from build123d import *

# Parameters (mm, degrees)
SKETCH1_R           = 14.125
BOSS_EXTRUDE1_DEPTH = 1.55
BOSS_EXTRUDE2_DEPTH = 1.55
SKETCH4_R           = 1.75
BOSS_EXTRUDE3_DEPTH = 9
CUT_EXTRUDE1_REACH  = 28.959
SKETCH5_R           = 4.75


with BuildPart() as part:
    # Sketch1 → Boss-Extrude1 (new body)
    with BuildSketch(Plane.XY):
        with Locations(Location((0, 0, 0), (0, 0, 180))):
            Circle(SKETCH1_R)
    extrude(amount=BOSS_EXTRUDE1_DEPTH)

    # Sketch2 → Boss-Extrude2 (add)
    with BuildSketch(Plane.XY):
        with BuildLine():
            Line((-17.5, 3.625), (17.5, 3.625))
            ThreePointArc((17.5, 3.625), (21.125, 0), (17.5, -3.625))
            Line((17.5, -3.625), (-17.5, -3.625))
            ThreePointArc((-17.5, -3.625), (-21.125, 0), (-17.5, 3.625))
        make_face()
    extrude(amount=BOSS_EXTRUDE2_DEPTH)

    # Sketch4 → Boss-Extrude3 (add)
    with BuildSketch(Plane.XY):
        with Locations((-17.5, 0)):
            Circle(SKETCH4_R)
        with Locations((17.5, 0)):
            Circle(SKETCH4_R)
    extrude(amount=BOSS_EXTRUDE3_DEPTH)

    # Sketch5 → Cut-Extrude1 (cut, up to next)
    with BuildSketch(Plane(origin=(0, 0, 0), x_dir=(-1, 0, 0), z_dir=(0, 0, -1)), mode=Mode.PRIVATE) as cut_extrude1_sk1:
        with Locations((0, 8)):
            Circle(SKETCH5_R)
    cut_extrude1_tool1 = extrude(cut_extrude1_sk1.sketch, amount=-CUT_EXTRUDE1_REACH, mode=Mode.PRIVATE) & part.part
    add(cut_extrude1_tool1.solids().sort_by_distance((0, 8, 0))[0], mode=Mode.SUBTRACT)


solid = part.part
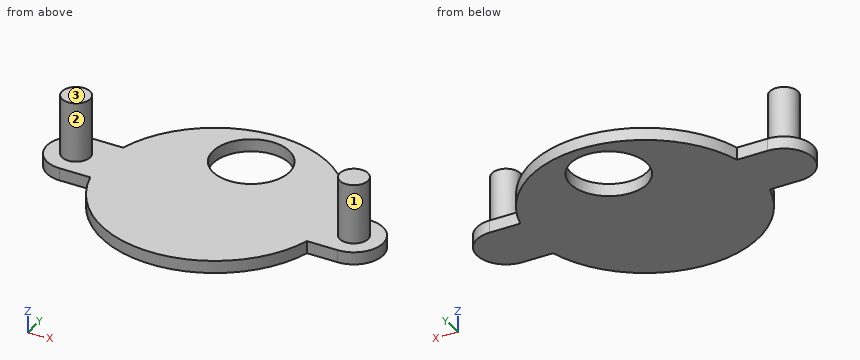
Part model, mm, in its own coordinate system. Face numbers are marked on the shaded views. Give positions to 0.01 mm unless a question says otherwise; leave off trailing zeros. Loops run counter-clockwise (first coordinate to the right, second up) from the corner with the lowest first, then second, coordinate; pieces in that order, holes last. Notation, with made-up numbers: M 57.25,87 L 73.25,87 A18 ccw 73.25,98 Z; hole C 23,40.5 d7. An arc over 180 degrees is marked long. Put each result on its own line as item: value. Start each with the question number.
1) Saw through at B-B (z = 1). List the corners of the cut face in (x, y) (3 decimals), then the cut area to 3 significant figures.
2) Saw through at C-C (y = 0). List the corners of the cut face in (x, z) (3 decimals), then the cut area to 3 significant figures.
3) Pull direction X, two halves, no side cores. Call the marked faces 1, 2 and 3: +X half, -X half, draft (parallel to the pull), parting line (faces both ways), or undercut.
4) Flat gauge pins, fed straight in: pin 1 (1.5 mm diameter, centred on y = 2, z = 3.5, fed in from +X); pin 2 (1.7 mm diameter, centred on x = -15, z = 1, fed in from -Y) (3 decimals); pin 3 (1.2 mm diameter, centred on x = 15, z = 0.5, fed in from +Y) (3 decimals); pin 4 (2 mm diameter, centred on x = -6, y = -7.5, fed in from -Z). Where does each tip first touch, or does it go through?
5) Saw through at D-D (y = 12). List the corners of the cut face in (x, z).
6) Saw through at A-A (x = 0). List the corners of the cut face in (y, z) (3 decimals).
7) Probe probe 1 along Z at (x, y) = (2.5, -12); probe 2 along X at (y, z) = (0.75, 7); probe 3 along X at (y, z) = (-0.5, 2.5). List the from-to ranges inside material, lowest first.
Numbers:
1. outline: M -17.5,-3.625 L -13.652,-3.625 A14.125 ccw 13.652,-3.625 L 17.5,-3.625 A3.625 ccw 17.5,3.625 L 13.652,3.625 A14.125 ccw -13.652,3.625 L -17.5,3.625 A3.625 ccw Z; hole C 0,8 d9.5
1. area: 648 mm^2
2. outline: M -21.125,0 L 21.125,0 L 21.125,1.55 L 19.25,1.55 L 19.25,9 L 15.75,9 L 15.75,1.55 L -15.75,1.55 L -15.75,9 L -19.25,9 L -19.25,1.55 L -21.125,1.55 Z
2. area: 118 mm^2
3. face 1: undercut
3. face 2: undercut
3. face 3: draft
4. pin 1: x = 18.72
4. pin 2: y = -3.625
4. pin 3: y = 3.625
4. pin 4: z = 0
5. outline: M -7.45,0 L -2.56,0 L -2.56,1.55 L -7.45,1.55 Z; M 2.56,0 L 7.45,0 L 7.45,1.55 L 2.56,1.55 Z
6. outline: M -14.125,0 L 3.25,0 L 3.25,1.55 L -14.125,1.55 Z; M 12.75,0 L 14.125,0 L 14.125,1.55 L 12.75,1.55 Z
7. probe 1: 0 to 1.55
7. probe 2: -19.08 to -15.92, 15.92 to 19.08
7. probe 3: -19.18 to -15.82, 15.82 to 19.18
